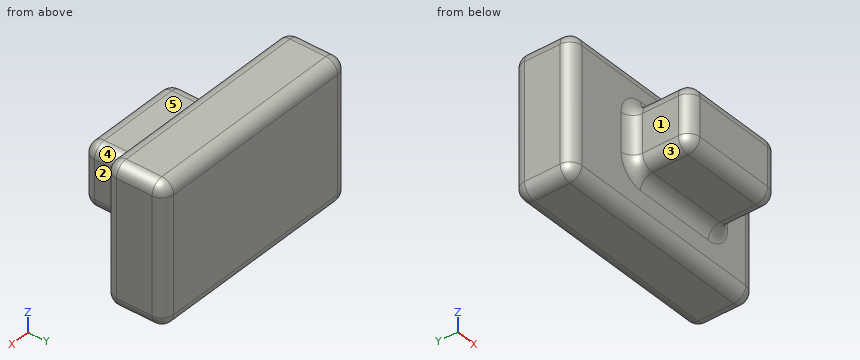
from build123d import *

# Parameters (mm, degrees)
F0_W     = 95.7648605108
F0_H     = 59.7243234515
F1_DEPTH = 25.4
F2_W     = 45.5140545964
F2_H     = 26.5670269728
F3_DEPTH = 50.8
F4_R     = 5.08


with BuildPart() as f1:
    # F0 (on Front) → F1 (new body)
    with BuildSketch(Plane.XZ):
        with Locations((0.8455961943, -4.4281929731)):
            Rectangle(F0_W, F0_H)
    extrude(amount=F1_DEPTH)

    # F2 (on Front) → F3 (join)
    with BuildSketch(Plane.XZ):
        with Locations((6.4061377198, -3.5014376044)):
            Rectangle(F2_W, F2_H)
    extrude(amount=F3_DEPTH)

    # F4
    f4_edges = [f1.edges().sort_by_distance(p)[0] for p in [
        (-16.35089, -38.1, -16.784951),
        (29.163165, -38.1, -16.784951),
        (48.728026, -12.7, -34.290355),
        (-47.036834, -12.7, -34.290355),
        (48.728026, -12.7, 25.433969),
        (29.163165, -38.1, 9.782076),
        (-47.036834, -12.7, 25.433969),
        (-16.35089, -38.1, 9.782076),
        (6.406138, -50.8, 9.782076),
        (6.406138, -50.8, -16.784951),
        (0.845596, -25.4, 25.433969),
        (-47.036834, -25.4, -4.428193),
        (0.845596, -25.4, -34.290355),
        (-47.036834, 0, -4.428193),
        (48.728026, 0, -4.428193),
        (0.845596, 0, -34.290355),
        (0.845596, 0, 25.433969),
        (48.728026, -25.4, -4.428193),
        (29.163165, -50.8, -3.501438),
        (6.406138, -25.4, -16.784951),
        (29.163165, -25.4, -3.501438),
        (-16.35089, -50.8, -3.501438),
        (6.406138, -25.4, 9.782076),
        (-16.35089, -25.4, -3.501438),
    ]]
    fillet(f4_edges, radius=F4_R)


solid = f1.part
The listing builds one solid part. Answer for the finished solid, in the listing's coordinates (mm). Face numbers are marked on the shaded views. A direction names the side the tool comes from. Give positions to 0.01 mm unless a question says otherwise; leave off trailing zeros. Loops run counter-clockwise (first coordinate to the right, second up) from the corner with the lowest first, then second, coordinate; pieces in that order, holes last.
Item 1: A cutting plane is placed at C-C (y = -32). Give the vertices of the cut face in (x, z).
Derived:
outline: (-16.35, -11.7) arc R5.08 ccw to (-11.27, -16.78) - (24.08, -16.78) arc R5.08 ccw to (29.16, -11.7) - (29.16, 4.7) arc R5.08 ccw to (24.08, 9.78) - (-11.27, 9.78) arc R5.08 ccw to (-16.35, 4.7) - close
Item 2: A cutting plane is placed at A-A (x = -33.5). Give the vertices of the cut face in (y, z), then the cut area to 3 significant figures.
Derived:
outline: (-25.4, -29.21) arc R5.08 ccw to (-20.32, -34.29) - (-5.08, -34.29) arc R5.08 ccw to (0, -29.21) - (0, 20.35) arc R5.08 ccw to (-5.08, 25.43) - (-20.32, 25.43) arc R5.08 ccw to (-25.4, 20.35) - close
area: 1,490 mm2
Item 3: Find the intervals of material crossed by line 1 along Y through (x, z) = (-37.5, -9); line 2 along Z through (x, y) = (-7, -39.5); line 3 along X through (y, z) = (-42.5, 2), in increasing order.
Derived:
line 1: y = -25.4 to 0
line 2: z = -16.78 to 9.78
line 3: x = -16.35 to 29.16
Item 4: Each of these flat-tipped pins is pushed along its axis until it touches: pin 1 Ø4.5 at (x, y) = (14, -35.5) entering from +Z; pin 2 Ø4.5 at (y, z) = (-41, -6.5) entering from +X; pin 3 Ø17 at (y, z) = (-41.5, -6) entering from -X; pin 4 Ø10 at (x, z) = (-15.5, -8) entering from -Y. Where does it stop, or does it pass through?
Derived:
pin 1: stops at z = 9.78
pin 2: stops at x = 29.16
pin 3: stops at x = -16.35
pin 4: stops at y = -50.8
Item 5: A cutting plane is placed at B-B (z = -9.5). Give the vertices of the cut face in (x, y).
Derived:
outline: (-47.04, -20.32) arc R5.08 ccw to (-41.96, -25.4) - (-21.43, -25.4) arc R5.08 cw to (-16.35, -30.48) - (-16.35, -45.72) arc R5.08 ccw to (-11.27, -50.8) - (24.08, -50.8) arc R5.08 ccw to (29.16, -45.72) - (29.16, -30.48) arc R5.08 cw to (34.24, -25.4) - (43.65, -25.4) arc R5.08 ccw to (48.73, -20.32) - (48.73, -5.08) arc R5.08 ccw to (43.65, 0) - (-41.96, 0) arc R5.08 ccw to (-47.04, -5.08) - close
Item 6: A cutting plane is placed at D-D (x = 23). Give the vertices of the cut face in (y, z), then the cut area to 3 significant figures.
Derived:
outline: (-50.8, -11.7) arc R5.08 ccw to (-45.72, -16.78) - (-30.48, -16.78) arc R5.08 cw to (-25.4, -21.86) - (-25.4, -29.21) arc R5.08 ccw to (-20.32, -34.29) - (-5.08, -34.29) arc R5.08 ccw to (0, -29.21) - (0, 20.35) arc R5.08 ccw to (-5.08, 25.43) - (-20.32, 25.43) arc R5.08 ccw to (-25.4, 20.35) - (-25.4, 14.86) arc R5.08 cw to (-30.48, 9.78) - (-45.72, 9.78) arc R5.08 ccw to (-50.8, 4.7) - close
area: 2,170 mm2
Item 7: A tool of negligible diameter and unlimited length cuts with its end or side. For the marked faces 1, 2, 3, 4 and 5, from which of +Z, -Z, +X, -X, +Y, -Y can it reach the whole face along a straight path? Write none if from no direction.
Derived:
face 1: +Z, -Z, -X, -Y
face 2: +Z, -Z, +X, -Y
face 3: -Z, -X, -Y
face 4: +Z, +X, -Y
face 5: +Z, +X, -X, -Y
